Verification items for the finished model (mm, model axes). Give positions to 0.01 mm unless a question says otherwise; leave off trailing zeros. Loops run counter-clockwise (first coordinate to the right, second up) from the corner with the lowest first, then second, coordinate; pieces in that order, holes last. Notation, with made-up numbers: (31.5, 5) -> (88.5, 5) arc R22 cw to (88.5, 25) -> close; hole circle Ø5 at (54.5, 22.25). An arc over 180 degrees is marked (long way). Answer in a Markdown table with one row per item. Add a question column.
Q1. Material ranges on probe 1 along Y at (x, z) = (79, 1.4); probe 2 along Y at (x, z) = (127.5, 0.55), recorded low to high.
Q2. Section check C-C on y = 153. Enter the section's corners in (x, z).
Q3. Section check A-A on y = 4. Enter the section's corners in (x, z), and give its area (3 significant figures).
Q4. Section check B-B on x = 79. Enter the section's corners in (y, z).
Q5. Gauge pin test, flat ends, axial feed: P1, Ø6.5, axis at x = 25, y = 45, coming from the -Z side; P2, Ø4.5, axis at x = 73.3, y = 4, coming from the -Z side. Record the tip position at first contact, or that the pin passes through.
```python
from build123d import *

# Parameters (mm, degrees)
SKETCH_1_W          = 146.6
SKETCH_1_H          = 200
EXTRUDE_1_DEPTH     = 1.5
SKETCH_2_R          = 2
CUT_EXTRUDE_1_DEPTH = 248.979454794
SKETCH_3_R          = 2
CUT_EXTRUDE_2_DEPTH = 248.979454794
SKETCH_4_R          = 2
CUT_EXTRUDE_3_DEPTH = 248.979454794
CHAMFER_1_SIZE      = 1.4


with BuildPart() as part:
    # Эскиз1 → Бобышка-Вытянуть1 (new body)
    with BuildSketch(Plane.XY):
        with Locations((73.3, 100)):
            Rectangle(SKETCH_1_W, SKETCH_1_H)
    extrude(amount=EXTRUDE_1_DEPTH)

    # Эскиз2 → Вырез-Вытянуть1 (cut, through all)
    with BuildSketch(Plane.XY.offset(1.5)):
        with Locations((20, 4)):
            Circle(SKETCH_2_R)
        with Locations((20, 196.5)):
            Circle(SKETCH_2_R)
        with Locations((73.3, 196.5)):
            Circle(SKETCH_2_R)
        with Locations((73.3, 4)):
            Circle(SKETCH_2_R)
        with Locations((126.6, 196.5)):
            Circle(SKETCH_2_R)
        with Locations((126.6, 4)):
            Circle(SKETCH_2_R)
    extrude(amount=-CUT_EXTRUDE_1_DEPTH, mode=Mode.SUBTRACT)

    # Эскиз3 → Вырез-Вытянуть2 (cut, through all)
    with BuildSketch(Plane.XY.offset(1.5)):
        with Locations((25, 45)):
            Circle(SKETCH_3_R)
        with Locations((79, 45)):
            Circle(SKETCH_3_R)
        with Locations((79, 129)):
            Circle(SKETCH_3_R)
        with Locations((25, 129)):
            Circle(SKETCH_3_R)
    extrude(amount=-CUT_EXTRUDE_2_DEPTH, mode=Mode.SUBTRACT)

    # Эскиз4 → Вырез-Вытянуть3 (cut, through all)
    with BuildSketch(Plane.XY.offset(1.5)):
        with Locations((116.6, 45)):
            Circle(SKETCH_4_R)
        with Locations((116.6, 153)):
            Circle(SKETCH_4_R)
    extrude(amount=-CUT_EXTRUDE_3_DEPTH, mode=Mode.SUBTRACT)

    # Фаска1
    chamfer_1_edges = [part.edges().sort_by_distance(p)[0] for p in [
        (124.6, 4, 0),
        (71.3, 196.5, 0),
        (71.3, 4, 0),
        (18, 196.5, 0),
        (124.6, 196.5, 0),
        (18, 4, 0),
        (23, 129, 0),
        (77, 129, 0),
        (77, 45, 0),
        (23, 45, 0),
        (114.6, 45, 0),
        (114.6, 153, 0),
    ]]
    chamfer(chamfer_1_edges, length=CHAMFER_1_SIZE)


solid = part.part
```
Taken from the geometry:
| question | item | result |
|---|---|---|
| 1 | probe 1 | y = 0 to 43, 47 to 127, 131 to 200 |
| 1 | probe 2 | y = 0 to 1.3, 6.7 to 193.8, 199.2 to 200 |
| 2 | outline | (0, 0) -> (113.2, 0) -> (114.6, 1.4) -> (114.6, 1.5) -> (0, 1.5) -> close; (118.6, 1.4) -> (120, 0) -> (146.6, 0) -> (146.6, 1.5) -> (118.6, 1.5) -> close |
| 3 | outline | (0, 0) -> (16.6, 0) -> (18, 1.4) -> (18, 1.5) -> (0, 1.5) -> close; (22, 1.4) -> (23.4, 0) -> (69.9, 0) -> (71.3, 1.4) -> (71.3, 1.5) -> (22, 1.5) -> close; (75.3, 1.4) -> (76.7, 0) -> (123.2, 0) -> (124.6, 1.4) -> (124.6, 1.5) -> (75.3, 1.5) -> close; (128.6, 1.4) -> (130, 0) -> (146.6, 0) -> (146.6, 1.5) -> (128.6, 1.5) -> close |
| 3 | area | 196 mm² |
| 4 | outline | (0, 0) -> (41.6, 0) -> (43, 1.4) -> (43, 1.5) -> (0, 1.5) -> close; (47, 1.4) -> (48.4, 0) -> (125.6, 0) -> (127, 1.4) -> (127, 1.5) -> (47, 1.5) -> close; (131, 1.4) -> (132.4, 0) -> (200, 0) -> (200, 1.5) -> (131, 1.5) -> close |
| 5 | P1 | stops at z = 0.15 |
| 5 | P2 | stops at z = 1.15 |
